```python
from build123d import *


# Not quite as in the source:
# - a fillet or chamfer that OpenCascade refuses, or shapes differently, is made with other operations: its cross-section is extruded or revolved along the edge and cut away or added
# - the dataset's text gives a spline's control points without its knots; the knots are read off the source's solid


with BuildPart() as f1:
    # F0 (on Front) → F1 (revolve)
    with BuildSketch(Plane.XZ):
        with BuildLine():
            Line((0, 47.7505947651), (0, 0))
            Line((0, 0), (25.4, 0))
            Line((25.4, 0), (25.4, 2.54))
            Line((25.4, 2.54), (6.9873421453, 2.54))
            Line((6.9873421453, 2.54), (6.9873421453, 7.3809963651))
            Line((6.9873421453, 7.3809963651), (3.0508127529, 7.3809963651))
            Line((3.0508127529, 7.3809963651), (3.0508127529, 45.4809963651))
            add(Edge.make_bspline(
                [(3.0508127529, 45.4809963651), (9.8461281639, 48.8954375707), (21.7228349186, 54.8631247901), (28.2240876429, 65.9165943611), (31.5127213678, 78.4358206865), (33.6784171743, 103.0849392109), (28.386283274, 115.9113566716), (25.8480589837, 122.0631897449)],
                knots=[0, 0, 0, 0, 0.2177295257, 0.3805430023, 0.5507700364, 0.7845393886, 1, 1, 1, 1], degree=3))
            Line((25.8480589837, 122.0631897449), (23.5000647508, 121.0944157349))
            add(Edge.make_bspline(
                [(1.9104079551, 47.7505947651), (3.8610263285, 48.7307217125), (7.7368881371, 50.6784180709), (12.2259767295, 53.1394673421), (15.4202565252, 55.1450698166), (17.2113496311, 56.4137046376), (18.4985579441, 57.4361542965), (19.3831690783, 58.2033768453), (20.1915430594, 58.9776879327), (21.1841928439, 60.0273218326), (22.2759624919, 61.3698248404), (23.392344712, 63.0381272524), (24.353200167, 64.7712061983), (25.0530786649, 66.2746693843), (25.5687607147, 67.5124472772), (26.0517126553, 68.761934225), (26.8207352465, 71.0094584469), (27.5553728133, 73.8128228874), (28.1157522153, 76.6310441845), (28.4178367466, 78.3658990039), (28.7101517328, 80.190879424), (29.0504794951, 82.6183883543), (29.5115503692, 86.7396383327), (29.8033217447, 91.1030083431), (29.8407350232, 95.4791342687), (29.7215088128, 98.7091824899), (29.4842699418, 101.3065910758), (29.202697145, 103.2994868111), (28.8607016819, 105.2540587373), (28.3291470633, 107.6283352293), (27.2887198112, 111.3164298649), (25.6928207945, 115.7785494719), (24.236343262, 119.3099152425), (23.5000647508, 121.0944157349)],
                knots=[4e-10, 4e-10, 4e-10, 4e-10, 0.0625000004, 0.1250000003, 0.1562500003, 0.1875000003, 0.2031250003, 0.2187500003, 0.2343750003, 0.2500000003, 0.2812500003, 0.3125000003, 0.3437500003, 0.3750000002, 0.3906250002, 0.4062500002, 0.4375000002, 0.5000000002, 0.5312500002, 0.5468750002, 0.5625000002, 0.5937500002, 0.6250000001, 0.6875000001, 0.7187500001, 0.7500000001, 0.7812500001, 0.7968750001, 0.8125000001, 0.8437500001, 0.875, 0.9375, 1, 1, 1, 1], degree=3))
            Line((1.9104079551, 47.7505947651), (0, 47.7505947651))
        make_face()
    revolve(axis=Axis((0, 0, 23.8752973825), (0, 0, -1)))

    # F2: fillet of radius 4.826 on 1 edges, made by hand

    # F2_s1 → F2_t2 (revolve, cut)
    with BuildSketch(Plane.XZ):
        with BuildLine():
            ThreePointArc((6.9873421453, 2.6376728427), (5.8750236847, 5.7196925415), (3.0508127529, 7.3809963651))
            Line((3.0508127529, 7.3809963651), (6.9873421453, 7.3809963651))
            Line((6.9873421453, 7.3809963651), (6.9873421453, 2.6376728427))
        make_face()
    revolve(axis=Axis((0, 0, 7.3809963651), (0, 0, -1)), mode=Mode.SUBTRACT)

    # F3: fillet of radius 7.62 on 1 edges, made by hand

    # F3_s1 → F3_t2 (revolve, cut)
    with BuildSketch(Plane.XZ):
        with BuildLine():
            ThreePointArc((19.7203873372, 2.54), (22.8312393105, 1.8760764803), (25.4, 0))
            Line((25.4, 0), (25.4, 2.54))
            Line((25.4, 2.54), (19.7203873372, 2.54))
        make_face()
    revolve(axis=Axis((0, 0, 2.54), (0, 0, -1)), mode=Mode.SUBTRACT)

    # F4: fillet of radius 5.08 on 1 edges, made by hand

    # F4_s1 → F4_t2 (revolve, cut)
    with BuildSketch(Plane.XZ):
        with BuildLine():
            ThreePointArc((23.5001194129, 121.0948119824), (25.9427148586, 120.0585616678), (27.5299870338, 117.93237864))
            Line((27.5299870338, 117.93237864), (28.0024132618, 118.1195048845))
            ThreePointArc((28.0024132618, 118.1195048845), (27.1665806291, 120.1928354079), (26.3177840752, 122.2569966352))
            Line((26.3177840752, 122.2569966352), (25.6542520935, 122.5329148365))
            ThreePointArc((25.6542520935, 122.5329148365), (24.4803481858, 122.048566289), (23.5695588788, 121.5981815612))
            Line((23.5695588788, 121.5981815612), (23.5001194129, 121.0948119824))
        make_face()
    revolve(axis=Axis((0, 0, 122.0631897449), (0, 0, -1)), mode=Mode.SUBTRACT)


solid = f1.part
```
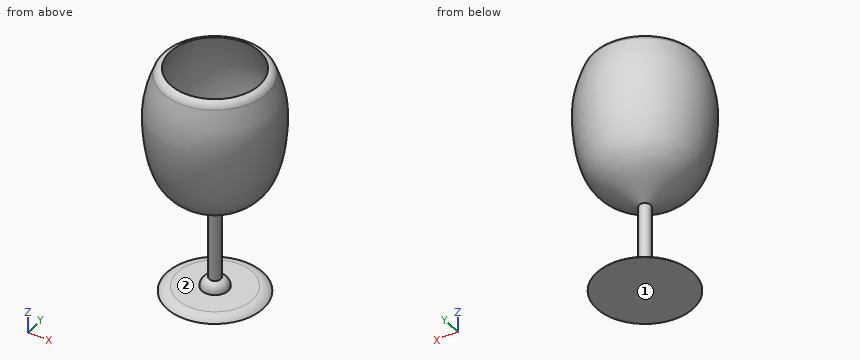
Input: part model. Units: mm. Frame: model coordinates. Face numbers are marked on the shaded views. A direction names the side the tool comes from. Coordinates: 2 decimals unless noted, no trailing zeros. Loops run counter-clockwise (first coordinate to the right, second up) from the corner with the lowest first, then second, coordinate; pieces in that order, holes last. Notation, with made-up numbers: M -15.5,71.25 L 31.5,71.25 A17 ccw 31.5,76.25 Z; hole C -39.75,4.25 d4. An arc over 180 degrees is marked long. Use a Markdown table: item, result. Add a question column.
1) Section A-A, the plane z = 27.5. Return the cut outline in (x, y).
2) Line query: L1, parallel to Z at x = -24, y = 4.5; L2, parallel to Z at x = 24, y = -6; L3, parallel to Y at x = -20, z = 78.5. Output: solid intervals per line, ascending. Write a range as from..to.
3) Set-up query: the marked faces 1 and 2. Return all of +Z, -Z, +X, -X, +Y, -Y with unobstructed straight access to the full face (end or side cutting, diameter ignored); none if empty.
4) Pin query (flat end, axial travel): P1, Ø5, axis at x = 24.5, z = 82, coming from the -Y side; P2, Ø3, axis at x = 11, y = -20, coming from the +Z side; P3, Ø4, axis at x = 23.5, z = 92, coming from the +Y side; P4, Ø10, axis at y = -12, z = 65, coming from the +X side. Return the tip coordinate at first contact, or that it passes through.
Answer below:
| question | item | result |
|---|---|---|
| 1 | outline | C 0,0 d6.1 |
| 2 | L1 | 0..0.92, 60.05..64.95, 118.86..120.88 |
| 2 | L2 | 0..0.65, 60.5..65.61, 118.07..120.76 |
| 2 | L3 | -23.7..-20.22, 20.22..23.7 |
| 3 | face 1 | -Z, +X, -X, +Y, -Y |
| 3 | face 2 | none |
| 4 | P1 | y = -22.61 |
| 4 | P2 | z = 121.09 |
| 4 | P3 | y = 24.14 |
| 4 | P4 | x = 27.38 |
